from build123d import *

# Parameters (mm, degrees)
AUFSATZ_LINEAR_AUSTRAGEN1_DEPTH = 3
SKIZZE2_R                       = 1.7
SCHNITT_LINEAR_AUSTRAGEN1_DEPTH = 57.435804238
DURCHGANGSLOCH_F_R_M41_D        = 4.5
DURCHGANGSLOCH_F_R_M31_D        = 3.4
VERRUNDUNG1_R                   = 2
SKIZZE9_W                       = 16
SKIZZE9_H                       = 17
SCHNITT_LINEAR_AUSTRAGEN2_DEPTH = 57.435804238


with BuildPart() as part:
    # Skizze1 → Aufsatz-Linear austragen1 (new body)
    with BuildSketch(Plane.XY):
        with BuildLine():
            Line((0, 0), (0, -9))
            Line((0, -9), (-5, -9))
            Line((-5, -9), (-5, -21))
            ThreePointArc((-5, -21), (-10, -26), (-15, -21))
            Line((-15, -21), (-15, -9))
            Line((-15, -9), (-20, -9))
            Line((-20, -9), (-20, 20))
            Line((-20, 20), (50, 20))
            Line((50, 20), (50, 0))
            Line((50, 0), (0, 0))
        make_face()
    extrude(amount=AUFSATZ_LINEAR_AUSTRAGEN1_DEPTH)

    # Skizze2 → Schnitt-Linear austragen1 (cut, through all)
    with BuildSketch(Plane.XY.offset(3)):
        with Locations((-10, -21)):
            Circle(SKIZZE2_R)
    extrude(amount=-SCHNITT_LINEAR_AUSTRAGEN1_DEPTH, mode=Mode.SUBTRACT)

    # Durchgangsloch für M41 (through all)
    with Locations(Plane.XY.offset(3)):
        with Locations((20, 10), (40, 10)):
            Hole(DURCHGANGSLOCH_F_R_M41_D / 2)

    # Durchgangsloch für M31 (through all)
    with Locations(Plane.XY.offset(3)):
        with Locations((-17.5, 12), (-2.5, -4), (-17.5, -4)):
            Hole(DURCHGANGSLOCH_F_R_M31_D / 2)

    # Verrundung1
    verrundung1_edges = [part.edges().sort_by_distance(p)[0] for p in [
        (0, 0, 1.5),
        (0, -9, 1.5),
        (-5, -9, 1.5),
        (-15, -9, 1.5),
        (-20, -9, 1.5),
        (-20, 20, 1.5),
        (50, 20, 1.5),
        (50, 0, 1.5),
    ]]
    fillet(verrundung1_edges, radius=VERRUNDUNG1_R)

    # Skizze9 → Schnitt-Linear austragen2 (cut, through all)
    with BuildSketch(Plane.XY.offset(3)):
        with Locations((-10, -17.5)):
            Rectangle(SKIZZE9_W, SKIZZE9_H)
    extrude(amount=-SCHNITT_LINEAR_AUSTRAGEN2_DEPTH, mode=Mode.SUBTRACT)


solid = part.part
Can you work these out from the model? Positions are in its coordinate system, mm. A direction names the side the tool comes from. Coordinates: 2 decimals unless noted, no trailing zeros. Write each loop counter-clockwise with the first axis right and the second up, starting at its lowest first coordinate (ties: lowest second). Pieces come first, ordered by that corner, then holes. Notation, with made-up numbers: (62, 11) - (79, 11) arc R11 ccw to (79, 23) - close; hole circle Ø4 at (-10, 49.5). An arc over 180 degrees is marked (long way). Return JSON: item names as keys, results as strings. Group by question number.
Item 1: If we section it at B-B (x = 40): Write out the boundary of the cut face in (y, z), then the cut area to 3 significant figures.
Item 2: We'd pull the mould along Y, two halves only. Please class faces 1 (the face through (-19.43, -8.4, 1.52)), 2 (the face through (-19.07, -4.65, 1.48)), 3 (the face through (42.248, 10.099, 1.479)), 4 (the face through (0, -4, 1)): pulls with the +Y half, pulls with the -Y half, needs draft (parallel to the pull), parting line crosses it, or undercut.
Item 3: Please list where these lines run through material, in increasing order: probe 1 along Y at (x, z) = (-2.5, 0.8); probe 2 along X at (y, z) = (-2.5, 0.6); probe 3 along Y at (x, z) = (40, 2.25).
Item 4: Which directions (+Z, -Z, +X, -X, +Y, -Y) give clear straight access to the entire face, cutting with the end or side of a thin tool? Please do faces 5 (the face through (-19.4, 19.43, 1.52)), 6 (the face through (25, 0, 1)).
Item 5: If we section it at A-A (y = -4): Write out the boundary of the cut face in (x, z), then the cut area to 3 significant figures.
Item 6: If we section it at C-C (z = 2.2): Write out the boundary of the cut face in (x, y).
Item 7: I'm going to push flat-ended pins straight in: pin 1 Ø5.5 at (x, y) = (-17.5, 12) entering from +Z; pin 2 Ø1 at (x, z) = (3.5, 1.5) entering from -Y; pin 3 Ø3.5 at (x, y) = (40, 10) entering from +Z. Where does each tip first touch, or does it pass through?
Item 8: If we section it at D-D (x = 5.5): Write out the boundary of the cut face in (y, z), then the cut area to 3 significant figures.
Return value:
{
 "1": {"outline": "(0, 0) - (7.75, 0) - (7.75, 3) - (0, 3) - close; (12.25, 0) - (20, 0) - (20, 3) - (12.25, 3) - close", "area": "46.5 mm^2"},
 "2": {"face 1": "pulls with the -Y half", "face 2": "undercut", "face 3": "undercut", "face 4": "needs draft"},
 "3": {"probe 1": "y = -9 to -5.7, -2.3 to 20", "probe 2": "x = -20 to -18.3, -16.7 to -3.3, -1.7 to 0", "probe 3": "y = 0 to 7.75, 12.25 to 20"},
 "4": {"face 5": "+Z, -Z, -X, +Y", "face 6": "+Z, -Z, +X, -Y"},
 "5": {"outline": "(-20, 0) - (-19.2, 0) - (-19.2, 3) - (-20, 3) - close; (-15.8, 0) - (-4.2, 0) - (-4.2, 3) - (-15.8, 3) - close; (-0.8, 0) - (0, 0) - (0, 3) - (-0.8, 3) - close", "area": "39.6 mm^2"},
 "6": {"outline": "(-20, -7) arc R2 ccw to (-18, -9) - (-2, -9) arc R2 ccw to (0, -7) - (0, -2) arc R2 cw to (2, 0) - (48, 0) arc R2 ccw to (50, 2) - (50, 18) arc R2 ccw to (48, 20) - (-18, 20) arc R2 ccw to (-20, 18) - close; hole circle Ø3.4 at (-17.5, -4); hole circle Ø3.4 at (-17.5, 12); hole circle Ø3.4 at (-2.5, -4); hole circle Ø4.5 at (20, 10); hole circle Ø4.5 at (40, 10)"},
 "7": {"pin 1": "stops at z = 3", "pin 2": "stops at y = 0", "pin 3": "passes through"},
 "8": {"outline": "(0, 0) - (20, 0) - (20, 3) - (0, 3) - close", "area": "60.0 mm^2"}
}
